from build123d import *

# Parameters (mm, degrees)
SKETCH2_R           = 1.5
BOSS_EXTRUDE1_DEPTH = 3
BOSS_EXTRUDE2_DEPTH = 60
SKETCH3_R           = 1.45
CUT_EXTRUDE1_DEPTH  = 10
CUT_EXTRUDE2_DEPTH  = 8
SKETCH5_R           = 2.5
CUT_EXTRUDE3_DEPTH  = 3
CHAMFER1_SIZE       = 1


with BuildPart() as part:
    # Sketch2 → Boss-Extrude1 (new body)
    # profile 1 of 3: a face of its own
    with BuildSketch(Plane(origin=(0, 0, 0), x_dir=(1, 0, 0), z_dir=(0, 1, 0))):
        Polygon((2.113248654, 0), (3.556624327, 2.5), (-3, 2.5), (-3, -2.5), (3.556624327, -2.5), align=None)
        with Locations(Location((0, 0, 0), (0, 0, 270))):
            Circle(SKETCH2_R, mode=Mode.SUBTRACT)
    # profile 2 of 3: a face of its own
    with BuildSketch(Plane(origin=(0, 0, 0), x_dir=(1, 0, 0), z_dir=(0, 1, 0))):
        Polygon((8, -2.5), (8, 2.5), (6.443375673, 2.5), (7.886751346, 0), (6.443375673, -2.5), align=None)
    # profile 3 of 3: a face of its own
    with BuildSketch(Plane(origin=(0, 0, 0), x_dir=(1, 0, 0), z_dir=(0, 1, 0))):
        Polygon((7.886751346, 0), (6.443375673, 2.5), (3.556624327, 2.5), (2.113248654, 0), (3.556624327, -2.5), (6.443375673, -2.5), align=None)
    extrude(amount=BOSS_EXTRUDE1_DEPTH)

    # Sketch2<3> → Boss-Extrude2 (add)
    with BuildSketch(Plane(origin=(0, 0, 0), x_dir=(1, 0, 0), z_dir=(0, 1, 0))):
        Polygon((3.556624327, 2.5), (2.113248654, 0), (3.556624327, -2.5), (6.443375673, -2.5), (7.886751346, 0), (6.443375673, 2.5), align=None)
    extrude(amount=BOSS_EXTRUDE2_DEPTH)

    # Sketch3 → Cut-Extrude1 (cut)
    with BuildSketch(Plane(origin=(0, 60, 0), x_dir=(1, 0, 0), z_dir=(0, 1, 0))):
        with Locations(Location((5, 0, 0), (0, 0, 270))):
            Circle(SKETCH3_R)
    extrude(amount=-CUT_EXTRUDE1_DEPTH, mode=Mode.SUBTRACT)

    # Sketch4 → Cut-Extrude2 (cut)
    with BuildSketch(Plane(origin=(0, 3, 0), x_dir=(1, 0, 0), z_dir=(0, 1, 0))):
        Polygon((6.443375673, 2.5), (8, 2.5), (8, -2.5), (6.443375673, -2.5), (7.886751346, 0), align=None)
    extrude(amount=-CUT_EXTRUDE2_DEPTH, mode=Mode.SUBTRACT)

    # Sketch5 → Cut-Extrude3 (cut)
    with BuildSketch(Plane(origin=(0, 3, 0), x_dir=(1, 0, 0), z_dir=(0, 1, 0))):
        Circle(SKETCH5_R)
    extrude(amount=CUT_EXTRUDE3_DEPTH, mode=Mode.SUBTRACT)

    # Chamfer1
    # the kernel refuses this chamfer: 1 mm, written as the material it takes off along each edge
    with BuildSketch(Plane(origin=(0.82740716, 6, -2.227142798), x_dir=(0.8656979742248804, -0.027495876610586487, -0.49981095845564805), z_dir=(0.4999999999999997, 0, 0.8660254037844388))) as chamfer1_piece_1_section:
        Polygon((CHAMFER1_SIZE * 0.999621916911, CHAMFER1_SIZE * 0.0274958766106), (-CHAMFER1_SIZE * 0.0274958766106, CHAMFER1_SIZE * 0.999621916911), (0, 0), align=None)
    chamfer1_piece_1 = extrude(amount=5.789866745, mode=Mode.PRIVATE)
    chamfer1_piece_1 = chamfer1_piece_1 & Plane(origin=(0, 6.406914482, 0), x_dir=(1, 0, 0), z_dir=(0, -1, 0)) * Cylinder(2.5, 16, mode=Mode.PRIVATE)
    add(chamfer1_piece_1, mode=Mode.SUBTRACT)
    with BuildSketch(Plane(origin=(3.722340533, 6, -2.787028888), x_dir=(0.8656979742248803, -0.027495876610586504, 0.4998109584556485), z_dir=(-0.5000000000000001, 0, 0.8660254037844386))) as chamfer1_piece_2_section:
        Polygon((CHAMFER1_SIZE * 0.999621916911, CHAMFER1_SIZE * 0.0274958766106), (-CHAMFER1_SIZE * 0.0274958766106, CHAMFER1_SIZE * 0.999621916911), (0, 0), align=None)
    chamfer1_piece_2 = extrude(amount=5.789866745, mode=Mode.PRIVATE)
    chamfer1_piece_2 = chamfer1_piece_2 & Plane(origin=(0, 6.406914482, 0), x_dir=(1, 0, 0), z_dir=(0, -1, 0)) * Cylinder(2.5, 16, mode=Mode.PRIVATE)
    add(chamfer1_piece_2, mode=Mode.SUBTRACT)


solid = part.part
Could you check a few things on this model? Use its own coordinates, in mm. A direction names the side the tool comes from. Give positions to 0.01 mm unless a question says otherwise; leave off trailing zeros. Order: outer loops, then holes, each group sorted by start corner. A loop starts at its lowest first (then second) coordinate and runs counter-clockwise, first axis right, second up.
Item 1: For faces 4 (the face through (2.845, 31.101, -1.267)), 5 (the face through (7.155, 30.42, 1.267)), 6 (the face through (5, 50, 0)), 7 (the face through (2.825, 31.101, 1.233)), 8 (the face through (4, 23, -2.5)), which set-ups out of +Z, -Z, +X, -X, +Y, -Y let a thin tool reach every point of the face, with its end or its side?
Item 2: I need wall thicknesses on line 1 (X direction, y = 1.55, z = 0); line 2 (Y direction, x = 2, z = -1.15); line 3 (Y direction, x = 4.75, z = 1.1). Which ranges of each line are inside material? Lowest first, please.
Item 3: If we section it at C-C, the plane x = 5: Write out the boundary of the cut face in (y, z), plus the area to 3 significant figures.
Item 4: If we section it at B-B, the plane y = 52: Write out the boundary of the cut face in (x, z).
Item 5: If we section it at A-A, the plane x = 0: Write out the boundary of the cut face in (y, z), plus the area to 3 significant figures.
Item 6: I'm going to push flat-ended pins straight in: pin 1 (1.5 mm diameter, centred on y = 30.5, z = 1, fed in from +X); pin 2 (2.5 mm diameter, centred on x = 1, z = -1, fed in from +Y); pin 3 (1 mm diameter, centred on y = 35.5, z = -1, fed in from +X). Where does each tip first touch, or does it pass through?
Item 7: If we section it at D-D, the plane y = 11: Write out the boundary of the cut face in (x, z), plus the area to 3 significant figures.
Item 8: If we mould it in two halves opening along Y, with no side actions, what happens to faces 1 (the face through (2, 0, 0)), 2 (the face through (0.45, 1.48, 1.43)), 3 (the face through (2.5, 5, 0))? For each: pulls with the +Y half, pulls with the -Y half, needs draft (parallel to the pull), parting line crosses it, or undercut.
Values:
1. face 4: -Z, -X, +Y
1. face 5: +Z, +X, +Y, -Y
1. face 6: +Y
1. face 7: +Z, -X, +Y
1. face 8: -Z, +X, -X, +Y, -Y
2. line 1: x = -3 to -1.5, 1.5 to 7.89
2. line 2: y = 0 to 3
2. line 3: y = 0 to 50
3. outline: (0, -2.5) - (60, -2.5) - (60, -1.45) - (50, -1.45) - (50, 1.45) - (60, 1.45) - (60, 2.5) - (0, 2.5) - close
3. area: 271 mm2
4. outline: (2.11, 0) - (3.56, -2.5) - (6.44, -2.5) - (7.89, 0) - (6.44, 2.5) - (3.56, 2.5) - close; hole circle Ø2.9 at (5, 0)
5. outline: (0, -2.5) - (3, -2.5) - (3, -1.5) - (0, -1.5) - close; (0, 1.5) - (3, 1.5) - (3, 2.5) - (0, 2.5) - close
5. area: 6.00 mm2
6. pin 1: stops at x = 7.74
6. pin 2: stops at y = 3
6. pin 3: stops at x = 7.6
7. outline: (2.11, 0) - (3.56, -2.5) - (6.44, -2.5) - (7.89, 0) - (6.44, 2.5) - (3.56, 2.5) - close
7. area: 21.7 mm2
8. face 1: pulls with the -Y half
8. face 2: needs draft
8. face 3: undercut
